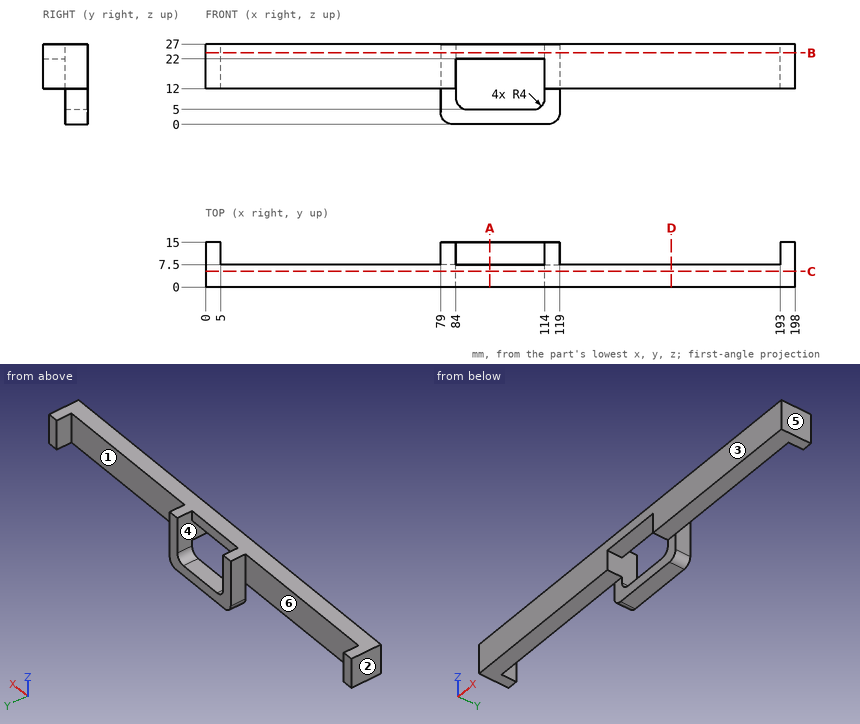
Source: three-view drawing plus pictorial views. Frame: mm from the lowest corner of the part. A direction names the side the tool comes from. Round coordinates to 2 decimals unless told otherwise and drop trailing zeros. Loops run counter-clockwise (first coordinate to the right, second up) from the corner with the lowest first, then second, coordinate; pieces in that order, holes last. Notation, with made-up numbers: M 17.5,-36.75 L 24.5,-36.75 A30 cw 24.5,-8.75 Z; hole C -17,78 d4. An arc over 180 degrees is marked long. Put each result on its own line as item: value.
(1) First-contact query: pin 1 (6 mm diameter, centred on x = 94.5, y = 3.5, fed in from -Z); pin 2 (12 mm diameter, centred on x = 147, z = 17, fed in from +Y); pin 3 (4.5 mm diameter, centred on x = 62, y = 11, fed in from -Z); pin 4 (4 mm diameter, centred on x = 104, y = 13, fed in from +Z). Flat tips, straight axial feed; report the tip coordinate or a pass-through.
Solutions:
pin 1: z = 22
pin 2: y = 7.5
pin 3: through
pin 4: z = 5
(2) Section D-D, the plane x = 156.5. Return loops of the section in (y, z), and give its area (4 significant figures).
Solutions:
outline: M 0,12 L 7.5,12 L 7.5,27 L 0,27 Z
area: 112.5 mm²
(3) Ray query, line 1 (X direction, y = 13, z = 16.5); line 2 (X direction, y = 3.75, z = 13.5); line 3 (Z direction, x = 71.5, y = 1). Return the intervals inside material, ascending. Write a range as [from, to].
Solutions:
line 1: [0, 5], [79, 84], [114, 119], [193, 198]
line 2: [0, 84], [114, 198]
line 3: [12, 27]
(4) Section B-B, the plane z = 24. Return loops of the section in (x, y), and give its area (4 significant figures).
Solutions:
outline: M 0,0 L 198,0 L 198,15 L 193,15 L 193,7.5 L 119,7.5 L 119,15 L 114,15 L 114,7.5 L 84,7.5 L 84,15 L 79,15 L 79,7.5 L 5,7.5 L 5,15 L 0,15 Z
area: 1,635 mm²
(5) Pull-direction query (X, two-part tool) for the marked faces 1, 2 and 3; classes: released by +X, released by -X, zero draft, split by the parting line, or undercut.
Solutions:
face 1: undercut
face 2: released by -X
face 3: zero draft
(6) Access query for the marked faces 4, 5 and 6. Directions: +Z, -Z, +X, -X, +Y, -Y. A direction counts if a zero-diameter tool reaches every point of the face in a straight line with its end or side. Return the directions, or none.
Solutions:
face 4: +Y
face 5: +Z, -Z, +X, +Y, -Y
face 6: +Z, -Z, +Y
(7) Section C-C, the plane y = 5.25. Return loops of the section in (x, z), and give its area (3 significant figures).
Solutions:
outline: M 0,12 L 84,12 L 84,22 L 114,22 L 114,12 L 198,12 L 198,27 L 0,27 Z
area: 2,670 mm²
(8) Section A-A, the plane x = 95.5. Return loops of the section in (y, z).
Solutions:
outline: M 0,22 L 7.5,22 L 7.5,27 L 0,27 Z; M 7.5,0 L 15,0 L 15,5 L 7.5,5 Z
